Design review of the part built by this model. Coordinates are the model's own, in mm. Face numbers are marked on the shaded views. A direction names the side the tool comes from. Give positions to 0.01 mm unless a question says otherwise; leave off trailing zeros. Write each loop counter-clockwise with the first axis right and the second up, starting at its lowest first coordinate (ties: lowest second). Pieces come first, ordered by that corner, then holes. Notation, with made-up numbers: M 64.5,38.25 L 74.5,38.25 A23 ccw 74.5,58.25 Z; hole C 7.5,71.25 d11. An arc over 180 degrees is marked long. Use one line per item in the form item = value. Start each with the question number.
from build123d import *

# Parameters (mm, degrees)
MAIN_DEPTH          = 10
BACKCUT_DEPTH       = 7
FILLET1_R           = 7
FIXHOLES_DEPTH      = 118.256129904
FIXHOLES_DEPTH_BACK = 118.256129904
SKETCH3_R           = 1.25


with BuildPart() as part:
    # Sketch1 → Main (new body)
    with BuildSketch(Plane.XY):
        with BuildLine():
            Line((-100, 0), (100, 0))
            Line((100, 0), (100, -30))
            Line((100, -30), (110, -40))
            Line((110, -40), (104.24709298, -40))
            ThreePointArc((104.24709298, -40), (71.998061986, -20), (39.749030993, -40))
            Line((39.749030993, -40), (32.249030993, -40))
            ThreePointArc((32.249030993, -40), (0, -20), (-32.249030993, -40))
            Line((-32.249030993, -40), (-39.749030993, -40))
            ThreePointArc((-39.749030993, -40), (-71.998061986, -20), (-104.24709298, -40))
            Line((-104.24709298, -40), (-110, -40))
            Line((-110, -40), (-100, -30))
            Line((-100, -30), (-100, 0))
        make_face()
    extrude(amount=MAIN_DEPTH)

    # Sketch2 → BackCut (cut)
    with BuildSketch(Plane.XY.offset(10)):
        with BuildLine():
            Line((-100, 0), (100, 0))
            Line((100, 0), (100, -22.534641377))
            Line((100, -22.534641377), (90, -22.534641377))
            ThreePointArc((90, -22.534641377), (62.748658295, -19.142863224), (40.327886742, -35))
            Line((40.327886742, -35), (31.670175244, -35))
            ThreePointArc((31.670175244, -35), (0, -18), (-31.670175244, -35))
            Line((-31.670175244, -35), (-40.327886742, -35))
            ThreePointArc((-40.327886742, -35), (-62.748658295, -19.142863224), (-90, -22.534641377))
            Line((-90, -22.534641377), (-100, -22.534641377))
            Line((-100, -22.534641377), (-100, 0))
        make_face()
    extrude(amount=-BACKCUT_DEPTH, mode=Mode.SUBTRACT)

    # Fillet1
    fillet1_edges = [part.edges().sort_by_distance(p)[0] for p in [
        (-62.748658295, -19.142863224, 3),
        (-95, -22.534641377, 3),
        (0, -18, 3),
        (95, -22.534641377, 3),
        (62.748658295, -19.142863224, 3),
        (-35.999030993, -35, 3),
        (35.999030993, -35, 3),
    ]]
    fillet(fillet1_edges, radius=FILLET1_R - 0.0001)  # a hair under: the kernel refuses the full size

    # Sketch3 → FixHoles (cut, two sides: drawn at the far end of the back side and taken through both)
    with BuildSketch(Plane.XY.offset(3).offset(-FIXHOLES_DEPTH_BACK)):
        with Locations((-45, -5)):
            Circle(SKETCH3_R)
        with Locations((45, -5)):
            Circle(SKETCH3_R)
        with Locations((-25, -15)):
            Circle(SKETCH3_R)
        with Locations((25, -15)):
            Circle(SKETCH3_R)
        with Locations((-85, -15)):
            Circle(SKETCH3_R)
        with Locations((85, -15)):
            Circle(SKETCH3_R)
    extrude(amount=FIXHOLES_DEPTH + FIXHOLES_DEPTH_BACK, mode=Mode.SUBTRACT)


solid = part.part
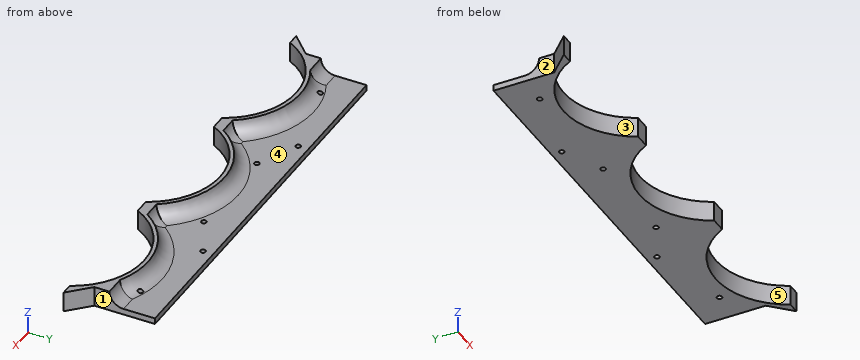
1. We need section A-A (z = 6.25). State the section outline as (x, y) points, and give its area (3 significant figures).
2. For the marked faces 4 and 5, list the 3-axis set-ups (+Z, -Z, +X, -X, +Y, -Y) from which the entire face can be reached by the end or side of a thin tool; tool diameter is ignored.
3. Clearance check with flat-ended pins moving along their axes: pin 1 Ø3 at (x, z) = (14, 6) entering from -Y; pin 2 Ø1.5 at (x, y) = (-25, -15) entering from +Z; pin 3 Ø3 at (x, y) = (45, -5) entering from +Z; pin 4 Ø3 at (x, y) = (85, -15) entering from +Z. State where each tip first meets the part, or that it passes through.
4. We need section B-B (y = -9). State the section outline as (x, z) points, and give its area (3 significant figures).
5. To check wall thickness, follow L1, parallel to X at y = -5, z = 2.3; L2, parallel to X at y = -15, z = 1.1; L3, parallel to X at y = -23, z = 8.5. State the ranges of each line that lie inside material, in increasing order.
6. Draft analysis for pull direction X (two halves, no side actions). For the marked faces 1, 2 and 3, state which applies: pulls with the +X half, pulls with the -X half, needs draft (parallel to the pull), parting line crosses it, or undercut.
Answer block:
q1.outline = M -110,-40 L -104.25,-40 A36 cw -39.75,-40 L -32.25,-40 A36 cw 32.25,-40 L 39.75,-40 A36 cw 104.25,-40 L 110,-40 L 100,-30 L 100,-21.45 L 90.27,-21.45 A39.09 ccw 39.75,-33.91 L 32.25,-33.91 A39.09 ccw -32.25,-33.91 L -39.75,-33.91 A39.09 ccw -90.27,-21.45 L -100,-21.45 L -100,-30 Z
q1.area = 899 mm^2
q2.face_4 = +Z, +Y
q2.face_5 = +Z, -Z, -Y
q3.pin_1 = -23.51
q3.pin_2 = through
q3.pin_3 = 3
q3.pin_4 = 3.93
q4.outline = M -100,0 L 100,0 L 100,3 L -100,3 Z
q4.area = 600 mm^2
q5.L1 = -100 to -46.25, -43.75 to 43.75, 46.25 to 100
q5.L2 = -100 to -86.25, -83.75 to -26.25, -23.75 to 23.75, 26.25 to 83.75, 86.25 to 100
q5.L3 = -100 to -86.39, -57.61 to -52.83, -19.17 to -14.39, 14.39 to 19.17, 52.83 to 57.61, 86.39 to 100
q6.face_1 = pulls with the +X half
q6.face_2 = pulls with the -X half
q6.face_3 = undercut
